from build123d import *

# Parameters (mm, degrees)
SKETCH1_W          = 10.2108
SKETCH1_H          = 18.7452
SKETCH2_R          = 4
CUT_EXTRUDE1_DEPTH = 9.525
CIRPATTERN1_COUNT  = 18
SKETCH4_R          = 6
CUT_EXTRUDE2_DEPTH = 9.525
FILLET1_R          = 6.35
SKETCH5_R          = 4
SKETCH5_R_2        = 27.94
SKETCH5_R_3        = 24.5
CUT_EXTRUDE3_DEPTH = 9.525


with BuildPart() as part:
    # Sketch1 → Revolve1 (revolve)
    with BuildSketch(Plane(origin=(0, 0, 0), x_dir=(0, 0, -1), z_dir=(1, 0, 0)), mode=Mode.PRIVATE) as revolve1_sk:
        with Locations((-82.1309, 9.3726)):
            Rectangle(SKETCH1_W, SKETCH1_H)
        Polygon((-77.0255, 18.7452), (-77.0255, 0), (-60.0329, 0), (-60.0329, 26.0096), (-77.0255, 26.0096), align=None)
        Polygon((-60.0329, 26.0096), (-60.0329, 0), (-56.5277, 0), (-56.5277, 45.9994), (-60.0329, 45.9994), align=None)
        Polygon((-56.5277, 45.9994), (-56.5277, 0), (29.4767, 0), (29.4767, 46.99), (29.4767, 113.5126), (-56.5277, 113.5126), align=None)
    revolve(revolve1_sk.sketch.rotate(Axis((0, 0, 87.2363), (0, 0, -1)), 180), axis=Axis((0, 0, 87.2363), (0, 0, -1)))

    # Sketch2 → Cut-Extrude1 (cut)
    with BuildSketch(Plane.XY.offset(60.0329)):
        with Locations((0, 39)):
            Circle(SKETCH2_R)
    cut_extrude1 = extrude(amount=-CUT_EXTRUDE1_DEPTH, mode=Mode.SUBTRACT)

    # CirPattern1: Cut-Extrude1 ×18 about axis, 2 skipped
    cirpattern1_axis = Axis((0, 0, 0), (0, 0, -1))
    add([cut_extrude1.rotate(cirpattern1_axis, i * 360 / CIRPATTERN1_COUNT) for i in range(1, CIRPATTERN1_COUNT) if i not in (8, 10)], mode=Mode.SUBTRACT)

    # Sketch4 → Cut-Extrude2 (cut)
    with BuildSketch(Plane.XY.offset(60.0329)):
        with Locations((-13.33878559, -36.648012211)):
            Circle(SKETCH4_R)
        with Locations((13.33878559, -36.648012211)):
            Circle(SKETCH4_R)
    extrude(amount=-CUT_EXTRUDE2_DEPTH, mode=Mode.SUBTRACT)

    # Fillet1
    fillet1_edges = [part.edges().sort_by_distance(p)[0] for p in [
        (0, 113.5126, 56.5277),
        (0, 113.5126, -29.4767),
    ]]
    fillet(fillet1_edges, radius=FILLET1_R)

    # Sketch5 → Cut-Extrude3 (cut)
    # profile 1 of 7: a face of its own
    with BuildSketch(Plane(origin=(0, 0, -29.4767), x_dir=(-1, 0, 0), z_dir=(0, 0, -1))):
        with Locations(Location((0, 37.5, 0), (0, 0, 90))):
            Circle(SKETCH5_R)
    # profile 2 of 7: a face of its own
    with BuildSketch(Plane(origin=(0, 0, -29.4767), x_dir=(-1, 0, 0), z_dir=(0, 0, -1))):
        with Locations(Location((32.475952642, 18.75, 0), (0, 0, 90))):
            Circle(SKETCH5_R)
    # profile 3 of 7: a face of its own
    with BuildSketch(Plane(origin=(0, 0, -29.4767), x_dir=(-1, 0, 0), z_dir=(0, 0, -1))):
        with Locations(Location((32.475952642, -18.75, 0), (0, 0, 90))):
            Circle(SKETCH5_R)
    # profile 4 of 7: a face of its own
    with BuildSketch(Plane(origin=(0, 0, -29.4767), x_dir=(-1, 0, 0), z_dir=(0, 0, -1))):
        with Locations(Location((0, -37.5, 0), (0, 0, 90))):
            Circle(SKETCH5_R)
    # profile 5 of 7: a face of its own
    with BuildSketch(Plane(origin=(0, 0, -29.4767), x_dir=(-1, 0, 0), z_dir=(0, 0, -1))):
        with Locations(Location((-32.475952642, -18.75, 0), (0, 0, 90))):
            Circle(SKETCH5_R)
    # profile 6 of 7: a face of its own
    with BuildSketch(Plane(origin=(0, 0, -29.4767), x_dir=(-1, 0, 0), z_dir=(0, 0, -1))):
        with Locations(Location((-32.475952642, 18.75, 0), (0, 0, 90))):
            Circle(SKETCH5_R)
    # profile 7 of 7: a face of its own
    with BuildSketch(Plane(origin=(0, 0, -29.4767), x_dir=(-1, 0, 0), z_dir=(0, 0, -1))):
        with Locations(Location((0, 0, 0), (0, 0, 90))):
            Circle(SKETCH5_R_2)
        with Locations(Location((0, 0, 0), (0, 0, 90))):
            Circle(SKETCH5_R_3, mode=Mode.SUBTRACT)
    extrude(amount=-CUT_EXTRUDE3_DEPTH, mode=Mode.SUBTRACT)


solid = part.part
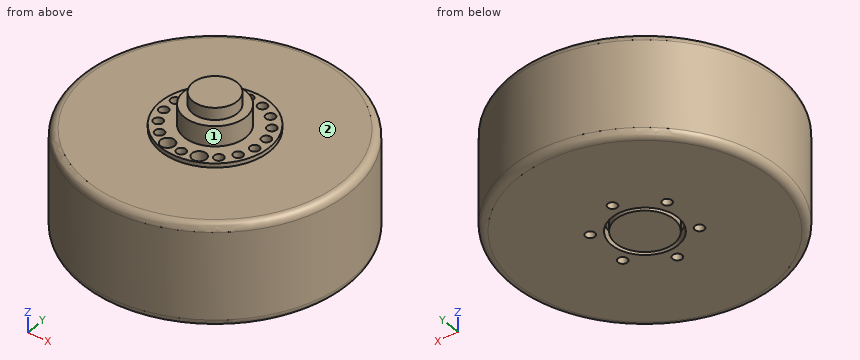
Can you work these out from the model? Positions are in its coordinate system, mm. Face numbers are marked on the shaded views. Coordinates: 2 decimals unless noted, no trailing zeros. Write each loop counter-clockwise with the first axis right and the second up, starting at its lowest first coordinate (ties: lowest second). Pieces come first, ordered by that corner, then holes. Notation, with made-up numbers: (32.5, 13.25) -> (68.5, 13.25) arc R14 ccw to (68.5, 39.25) -> close; hole circle Ø11 at (69.25, 29). An arc over 180 degrees is marked (long way). Write each question's results on one line, items separated by ' | '. Start each with the question number.
Item 1: If we section it at A-A, the plane z = 26.5: Write out the boundary of the cut face in (x, y).
Item 2: Thinking about a two-plate mould opening in Y: for the marked faces 1 and 2, which applies, released by +Y, released by -Y, zero draft, split by the parting line, or undercut?
Item 3: Please list where these lines run through material, in increasing order: probe 1 along X at (y, z) = (0, -24.5); probe 2 along Z at (x, y) = (17.5, 49); probe 3 along Y at (x, z) = (33, 51).
Item 4: I'm going to push flat-ended pins straight in: P1, Ø9, axis at x = 0, y = 39, coming from the +Z side; P2, Ø6, axis at x = -54.5, z = 55.5, coming from the -Y side; P3, Ø6, axis at x = 37.5, z = 9.5, coming from the -Y side. Where does each tip first touch, or does it pass through?
Answer block:
1) outline: circle Ø227.03 at (0, 0)
2) face 1: split by the parting line | face 2: zero draft
3) probe 1: -113.36 to -27.94, -24.5 to 24.5, 27.94 to 113.36 | probe 2: -29.48 to 56.53 | probe 3: -108.55 to -23.42, -15.58 to 15.58, 23.42 to 108.55
4) P1: z = 60.03 | P2: y = -99.74 | P3: y = -108.14
